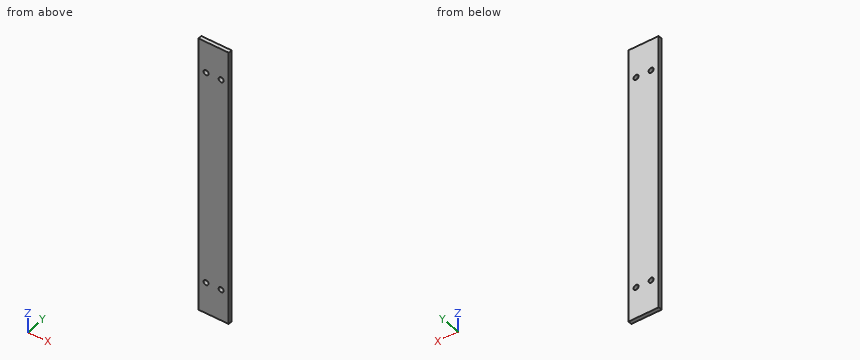
Autodesk Inventor part; units mm, degrees
ref_plane "YZ Plane" through (0, 0, 0) normal (1, 0, 0) x (0, 1, 0)
ref_plane "XZ Plane" through (0, 0, 0) normal (0, 1, 0) x (-1, 0, 0)
ref_plane "XY Plane" through (0, 0, 0) normal (0, 0, 1) x (1, 0, 0)
sketch "Sketch1" plane through (0, 0, 0) normal (0, 1, 0) x (-1, 0, 0)
  line L0 (-12, 110.5) -> (12, 110.5)
  line L1 (12, 110.5) -> (12, -110.5)
  line L2 (12, -110.5) -> (-12, -110.5)
  line L3 (-12, -110.5) -> (-12, 110.5)
  line L4 (-12, 110.5) -> (12, -110.5) construction
  line L5 (12, 110.5) -> (-12, -110.5) construction
  point P0 (0, 0)
  dimension "d0" = 24
  dimension "d1" = 221
extrude "Extrusion1" add sketch "Sketch1" along normal blind 3
sketch "Sketch2" plane through (0, 3, 0) normal (0, 1, 0) x (1, 0, 0)
  line L0 (12, -110.5) -> (12, 110.5)
  line L1 (-12, -110.5) -> (12, -110.5)
  point P0 (0, 0)
  point P1 (-6, -85.5)
  point P2 (6, -85.5)
  point P3 (-6, 85.5)
  point P4 (6, 85.5)
  dimension "d4" = 12
  dimension "d5" = 6
  dimension "d6" = 171
  dimension "d7" = 25
hole "Hole1" at (-6, 3, 85.5) at (6, 3, 85.5) at (-6, 3, -85.5) at (6, 3, -85.5) direction (0, -1, 0) diameter 4 depth 3
properties part number "213"
CAD build for the part. Positions are in the model's coordinates, mm. Round coordinates to 2 decimals unless told otherwise and drop trailing zeros. Order: outer loops, then holes, each group sorted by start corner. A loop starts at its lowest first (then second) coordinate and runs counter-clockwise, first axis right, second up. Notation, with made-up numbers: (64, 16.5) - (90, 16.5) arc R17 cw to (90, 43.5) - close; hole circle Ø6 at (-13.5, 50.5). An arc over 180 degrees is marked (long way). Answer as CSV lines item,"result". Start each with the question number.
1. Pin check, flat tip, straight feed: pin 1 (1 mm diameter, centred on x = 4, z = -3.5, fed in from -Y). Stop position of the tip, or through.
2. Drill centre lines: L1, parallel to Z at x = -6, y = 0.7; L2, parallel to X at y = 1.65, z = -85.5; L3, parallel to Z at x = 4.5, y = 0.65. Where is each one in solid material? Low to high. Write a range as [from, to].
3. Saw through at A-A, the plane z = -85.5. Write the cut outline in (x, y).
4. Saw through at B-B, the plane x = -6. Write the cut outline in (y, z), and give its area (3 significant figures).
Model answer:
1,pin 1,"stops at y = 0"
2,L1,"z = [-110.5, -87.5], [-83.5, 83.5], [87.5, 110.5]"
2,L2,"x = [-12, -8], [-4, 4], [8, 12]"
2,L3,"z = [-110.5, -86.82], [-84.18, 84.18], [86.82, 110.5]"
3,outline,"(-12, 0) - (-8, 0) - (-8, 3) - (-12, 3) - close; (-4, 0) - (4, 0) - (4, 3) - (-4, 3) - close; (8, 0) - (12, 0) - (12, 3) - (8, 3) - close"
4,outline,"(0, -110.5) - (3, -110.5) - (3, -87.5) - (0, -87.5) - close; (0, -83.5) - (3, -83.5) - (3, 83.5) - (0, 83.5) - close; (0, 87.5) - (3, 87.5) - (3, 110.5) - (0, 110.5) - close"
4,area,"639 mm²"
